from build123d import *

# Parameters (mm, degrees)
F0_R          = 201.6125
F0_R_2        = 200.025
F1_DEPTH      = 2032
F2_W          = 25.4
F2_H          = 25.4
F3_DEPTH      = 508
F4_DEPTH      = 2714
F4_DEPTH_BACK = 709.6135
F5_W          = 25.4
F5_H          = 12.7
F6_DEPTH      = 201.6135
F6_DEPTH_BACK = 201.6135


# Not quite as in the source:
# - an extrude ends at something that could not be found from the text; its depth is read off the source's solid


with BuildPart() as f1:
    # F0 (on Right) → F1 (new body)
    with BuildSketch(Plane.YZ):
        Circle(F0_R)
        Circle(F0_R_2, mode=Mode.SUBTRACT)
    extrude(amount=F1_DEPTH)


with BuildPart() as f3:
    # F2 (on Top) → F3 (new body)
    with BuildSketch(Plane.XY):
        with Locations((812.8, 0)):
            Rectangle(F2_W, F2_H)
    extrude(amount=F3_DEPTH)


with BuildPart() as f4_tool:
    # F4 (cut, two sides): a face of the model
    f4_faces = [f3.part.faces().sort_by_distance(p)[0] for p in [
        (812.8, 0, 508),
    ]]
    extrude(f4_faces, amount=F4_DEPTH)
    extrude(f4_faces, amount=-F4_DEPTH_BACK)


with BuildPart() as f1_1:
    add(f1.part)

    # F4: cut by f4_tool
    add(f4_tool.part, mode=Mode.SUBTRACT)

    # F5 (on Top) → F6 (cut, two sides)
    with BuildSketch(Plane.XY) as f6_sk:
        with Locations((203.2, 0)):
            Rectangle(F5_W, F5_H)
        with Locations((609.6, 0)):
            Rectangle(F5_W, F5_H)
        with Locations((1016, 0)):
            Rectangle(F5_W, F5_H)
        with Locations((1422.4, 0)):
            Rectangle(F5_W, F5_H)
        with Locations((1828.8, 0)):
            Rectangle(F5_W, F5_H)
    extrude(amount=F6_DEPTH, mode=Mode.SUBTRACT)
    extrude(f6_sk.sketch, amount=-F6_DEPTH_BACK, mode=Mode.SUBTRACT)


with BuildPart() as f3_1:
    add(f3.part)

    # F4: cut by f4_tool
    add(f4_tool.part, mode=Mode.SUBTRACT)


solid = f1_1.part
Check sheet for the modelled part. Datum: model origin and axes. Units: mm. Round coordinates to 2 decimals unless told otherwise and drop trailing zeros. Order: outer loops, then holes, each group sorted by start corner. A loop starts at its lowest first (then second) coordinate and runs counter-clockwise, first axis right, second up.
Q1. Draft check along Y on faces 1 (the face through (1001.78, -159.99, -122.68)), 2 (the face through (1001.78, -43.36, -195.27)). Enter one of: pulls with the +Y half, pulls with the -Y half, needs draft (parallel to the pull), parting line crosses it, or undercut.
Filled sheet:
face 1: parting line crosses it
face 2: undercut
Q2. Scan lines: L1, parallel to Z at x = 1304.5, y = 0 (1 decimal); L2, parallel to Y at x = 1797, z = -6.5; L3, parallel to Y at x = 409.5, z = 9. Record each from-to range of solid material in increasing order.
Filled sheet:
L1: z = -201.6 to -200, 200 to 201.6
L2: y = -201.51 to -199.92, 199.92 to 201.51
L3: y = -201.41 to -199.82, 199.82 to 201.41
Q3. Cross-section at B-B, the plane y = 132. Enter the section's corners in (x, z).
Filled sheet:
outline: (0, -152.39) - (2032, -152.39) - (2032, -150.29) - (0, -150.29) - close; (0, 150.29) - (2032, 150.29) - (2032, 152.39) - (0, 152.39) - close
Q4. Depth check by flat-ended pin: P1, Ø12, axis at x = 1554.5, y = -79, coming from the -Z side; P2, Ø6, axis at x = 362, y = 83.5, coming from the -Z side; P3, Ø3, axis at x = 842.5, z = -110.5, coming from the -Y side. Enter the tip coordinate at first touch or a pass-through.
Filled sheet:
P1: stops at z = -187.93
P2: stops at z = -184.84
P3: stops at y = -169.61
Q5. Cross-section at A-A, the plane z = 0. Enter the section's corners in (x, y) (1 decimal), plus the area to 3 significant figures.
Filled sheet:
outline: (0, -201.6) - (2032, -201.6) - (2032, -200) - (0, -200) - close; (0, 200) - (2032, 200) - (2032, 201.6) - (0, 201.6) - close
area: 6,450 mm2
